The listing builds one solid part. Answer for the finished solid, in the listing's coordinates (mm). A direction names the side the tool comes from. Round coordinates to 2 decimals unless told otherwise and drop trailing zeros. Loops run counter-clockwise (first coordinate to the right, second up) from the corner with the lowest first, then second, coordinate; pieces in that order, holes last. Notation, with made-up numbers: (6.5, -25.5) -> (20.5, -25.5) arc R34 cw to (20.5, 13.5) -> close; hole circle Ø4 at (-24, 31.25). An arc over 180 degrees is marked (long way). One line per question, with ' | ' between items.
from build123d import *

# Parameters (mm, degrees)
SKETCH1_R           = 1.575
SKETCH1_R_2         = 1.5875
SKETCH1_R_3         = 1.75
BOSS_EXTRUDE1_DEPTH = 3
FILLET1_R           = 5


with BuildPart() as part:
    # Sketch1 → Boss-Extrude1 (new body)
    with BuildSketch(Plane.XY):
        with BuildLine():
            Line((-55, -3.774250665), (-33.235815946, -50.880076598))
            ThreePointArc((-33.235815946, -50.880076598), (-31.390782754, -52.995176633), (-28.696863862, -53.782956197))
            Line((-28.696863862, -53.782956197), (28.696863862, -53.782956197))
            ThreePointArc((28.696863862, -53.782956197), (31.390782754, -52.995176633), (33.235815946, -50.880076598))
            Line((33.235815946, -50.880076598), (55, -3.774250665))
            Line((55, -3.774250665), (55, 16.225749335))
            Line((55, 16.225749335), (40, 16.225749335))
            Line((40, 16.225749335), (40, 76.225749335))
            Line((40, 76.225749335), (-40, 76.225749335))
            Line((-40, 76.225749335), (-40, 16.225749335))
            Line((-40, 16.225749335), (-55, 16.225749335))
            Line((-55, 16.225749335), (-55, -3.774250665))
        make_face()
        with Locations((-37.673971089, -6.665090314)):
            Circle(SKETCH1_R, mode=Mode.SUBTRACT)
        with Locations((37.673971089, -6.665090314)):
            Circle(SKETCH1_R, mode=Mode.SUBTRACT)
        with Locations((32.208377558, 17.056918669)):
            Circle(SKETCH1_R_2, mode=Mode.SUBTRACT)
        with Locations((32.208377558, 44.996918669)):
            Circle(SKETCH1_R_2, mode=Mode.SUBTRACT)
        with Locations((-19.861622442, 11.976918669)):
            Circle(SKETCH1_R_2, mode=Mode.SUBTRACT)
        with Locations((-18.591622442, 60.236918669)):
            Circle(SKETCH1_R_2, mode=Mode.SUBTRACT)
        with Locations((-26.592001418, 67.180357374)):
            Circle(SKETCH1_R_3, mode=Mode.SUBTRACT)
        with Locations((26.592001418, 67.180357374)):
            Circle(SKETCH1_R_3, mode=Mode.SUBTRACT)
        with Locations((-18.75, -8.749633405)):
            Circle(SKETCH1_R, mode=Mode.SUBTRACT)
        with Locations((18.75, -8.749633405)):
            Circle(SKETCH1_R, mode=Mode.SUBTRACT)
        with Locations((-18.75, -46.249633405)):
            Circle(SKETCH1_R, mode=Mode.SUBTRACT)
        with Locations((18.75, -46.249633405)):
            Circle(SKETCH1_R, mode=Mode.SUBTRACT)
        Polygon((-41.411487692, -23.690735407), (-33.073456052, -19.802647399), (-26.90322943, -33.03474109), (-35.241261071, -36.922829098), align=None, mode=Mode.SUBTRACT)
        with BuildLine():
            Line((-41.63599241, -20.485289919), (-35.384660905, -17.570246165))
            ThreePointArc((-35.384660905, -17.570246165), (-34.90097138, -16.241320116), (-36.229897428, -15.757630591))
            Line((-36.229897428, -15.757630591), (-42.481228933, -18.672674345))
            ThreePointArc((-42.481228933, -18.672674345), (-42.964918459, -20.001600394), (-41.63599241, -20.485289919))
        make_face(mode=Mode.SUBTRACT)
    extrude(amount=BOSS_EXTRUDE1_DEPTH)

    # Fillet1
    fillet1_edges = [part.edges().sort_by_distance(p)[0] for p in [
        (-55, 16.225749335, 1.5),
        (-40, 16.225749335, 1.5),
        (-40, 76.225749335, 1.5),
        (40, 76.225749335, 1.5),
        (40, 16.225749335, 1.5),
        (55, 16.225749335, 1.5),
    ]]
    fillet(fillet1_edges, radius=FILLET1_R)


solid = part.part
Q1. A cutting plane is placed at B-B on y = -26.5. Give the vertices of the cut face in (x, z).
Numbers:
outline: (-44.5, 0) -> (-40.1, 0) -> (-40.1, 3) -> (-44.5, 3) -> close; (-29.95, 0) -> (44.5, 0) -> (44.5, 3) -> (-29.95, 3) -> close
Q2. Given pin 1 Ø4 at (x, y) = (-18.75, -46.25) entering from +Z; pin 2 Ø0.9 at (y, z) = (48, 2) entering from -X; pin 3 Ø1.5 at (x, z) = (47, 1) entering from +Y, each flat-ended and moving along its own axis, determine where each tip first touches the part or whether it passes through.
Numbers:
pin 1: z = 3 | pin 2: x = -40 | pin 3: y = 16.23
Q3. Find the intervals of material crossed by line 1 (Y direction, x = 18.75, z = 2.15); line 2 (Y direction, x = -19, z = 2.4); line 3 (X direction, y = -8.5, z = 2), in increasing order. Write a range as from..to.
Numbers:
line 1: -53.78..-47.82, -44.67..-10.32, -7.17..76.23 | line 2: -53.78..-47.8, -44.69..-10.3, -7.19..10.64, 13.31..58.7, 61.77..76.23 | line 3: -52.82..-20.31, -17.19..17.19, 20.31..52.82
Q4. A cutting plane is placed at D-D on z = 2.1. Give the number of separate pieces and of enclosed holes in the cut face, plus the area to 3 significant figures.
Numbers:
separate pieces: 1 | enclosed holes: 14 | area: 11,100 mm^2
Q5. For faces 4 (the face through (-40, 47, 1)), 5 (the face through (-1, 12, 0)), 6 (the face through (-31.01, -34.95, 1.48)), determine the directions among +Z, -Z, +X, -X, +Y, -Y from which every point of the face is accessible in a straight line to the end or side of a thin tool.
Numbers:
face 4: +Z, -Z, -X, +Y | face 5: -Z, +X, -X, +Y, -Y | face 6: +Z, -Z
Q6. A cutting plane is placed at C-C on y = 42. Give the vertices of the cut face in (x, z), plus the area to 3 significant figures.
Numbers:
outline: (-40, 0) -> (40, 0) -> (40, 3) -> (-40, 3) -> close | area: 240 mm^2
Q7. A cutting plane is placed at A-A on x = 18.75. Give the vertices of the cut face in (y, z).
Numbers:
outline: (-53.78, 0) -> (-47.82, 0) -> (-47.82, 3) -> (-53.78, 3) -> close; (-44.67, 0) -> (-10.32, 0) -> (-10.32, 3) -> (-44.67, 3) -> close; (-7.17, 0) -> (76.23, 0) -> (76.23, 3) -> (-7.17, 3) -> close
Q8. For a pull along Y with two mould halves and no side action, classify faces 1 (the face through (0, 76.226, 1)), 2 (the face through (-1, 12, 3)), 3 (the face through (-38.554, -19.048, 1.479)) as pulls with the +Y half, pulls with the -Y half, needs draft (parallel to the pull), parting line crosses it, or undercut.
Numbers:
face 1: pulls with the +Y half | face 2: needs draft | face 3: undercut
